Geometry: final body of the model. Coordinates: model frame, mm. A direction names the side the tool comes from. Coordinates: 2 decimals unless noted, no trailing zeros. Write each loop counter-clockwise with the first axis right and the second up, starting at its lowest first coordinate (ties: lowest second). Pieces come first, ordered by that corner, then holes. Notation, with made-up numbers: (-15, -21.75) - (-1, -21.75) arc R17 ccw to (-1, -17.75) - close; hole circle Ø9 at (19.25, 14). An arc over 180 degrees is marked (long way). Put each result on its own line as item: value.
```python
from build123d import *

# Parameters (mm, degrees)
F0_W     = 63.5
F0_H     = 63.5
F1_DEPTH = 63.5
F2_W     = 50.8
F2_H     = 50.8
F3_DEPTH = 57.15
F4_W     = 57.15
F4_H     = 57.15
F5_DEPTH = 59.69


with BuildPart() as f1:
    # F0 (on Top) → F1 (new body)
    with BuildSketch(Plane.XY):
        Rectangle(F0_W, F0_H)
    extrude(amount=F1_DEPTH)

    # F2 (on face) → F3 (cut)
    with BuildSketch(Plane.XZ.offset(31.75)):
        with Locations((0, 31.75)):
            Rectangle(F2_W, F2_H)
    extrude(amount=-F3_DEPTH, mode=Mode.SUBTRACT)

    # F4 (on face) → F5 (cut)
    with BuildSketch(Plane.XY.offset(63.5)):
        Rectangle(F4_W, F4_H)
    extrude(amount=-F5_DEPTH, mode=Mode.SUBTRACT)


solid = f1.part
```
1. Section query C-C (y = -14). Return loops of the section in (x, z) (3 decimals), then the cut area to 3 significant figures.
Answer below:
outline: (-31.75, 0) - (31.75, 0) - (31.75, 63.5) - (28.575, 63.5) - (28.575, 3.81) - (-28.575, 3.81) - (-28.575, 63.5) - (-31.75, 63.5) - close
area: 621 mm²
2. Pin query (flat end, axial travel): pin 1 Ø3 at (x, z) = (19, 51) entering from -Y (3 decimals); pin 2 Ø12 at (x, y) = (-13, 21) entering from +Z. Return the tip coordinate at first contact, or that it passes through.
Answer below:
pin 1: stops at y = 28.575
pin 2: stops at z = 3.81
3. Ray query, probe 1 along X at (y, z) = (-16, 12.5) (3 decimals); probe 2 along Z at (x, y) = (-5, -17). Return the intervals inside material, ascending. Write a range as from..to.
Answer below:
probe 1: x = -31.75..-28.575, 28.575..31.75
probe 2: z = 0..3.81
4. Mould query, pull axis Y, two halves, no side actions, for faces 1 (the flat face through (0, 0, 3.81)), 2 (the flat face through (0, -30, 57.15)), 3 (the flat face through (-29, -31.75, 31)). Classes: +Y half, -Y half, draft (parallel to the pull), parting line (faces both ways), or undercut.
Answer below:
face 1: undercut
face 2: draft
face 3: -Y half
5. Set-up query: faces 4 (the flat face through (25.4, -30, 31)), 5 (the flat face through (-28.575, 0, 34)), 6 (the flat face through (0, 0, 0)). Return all of +Z, -Z, +X, -X, +Y, -Y with unobstructed straight access to the full face (end or side cutting, diameter ignored); none if empty.
Answer below:
face 4: -Y
face 5: +Z
face 6: -Z, +X, -X, +Y, -Y
6. Section query B-B (x = 10). Return loops of the section in (y, z) (3 decimals).
Answer below:
outline: (-31.75, 0) - (31.75, 0) - (31.75, 63.5) - (28.575, 63.5) - (28.575, 3.81) - (-28.575, 3.81) - (-28.575, 6.35) - (-31.75, 6.35) - close; (-31.75, 57.15) - (-28.575, 57.15) - (-28.575, 63.5) - (-31.75, 63.5) - close
7. Section query A-A (z = 49.5). Return loops of the section in (x, y) (3 decimals), then the cut area to 3 significant figures.
Answer below:
outline: (-31.75, -31.75) - (-25.4, -31.75) - (-25.4, -28.575) - (-28.575, -28.575) - (-28.575, 28.575) - (28.575, 28.575) - (28.575, -28.575) - (25.4, -28.575) - (25.4, -31.75) - (31.75, -31.75) - (31.75, 31.75) - (-31.75, 31.75) - close
area: 605 mm²
